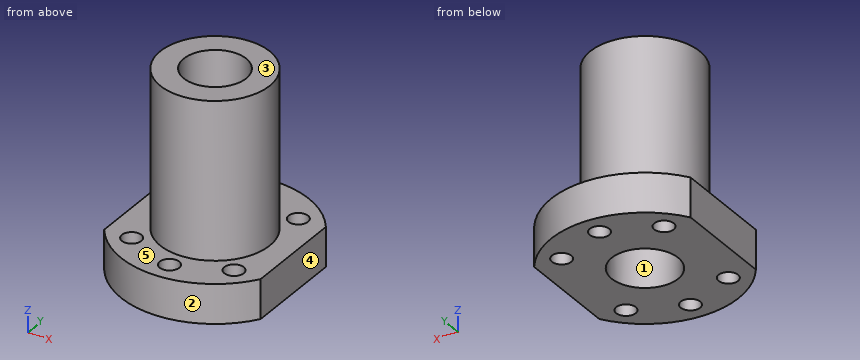
```python
from build123d import *

# Parameters (mm, degrees)
SKETCH_R      = 2.5
SKETCH_R_2    = 8.5
PAD_DEPTH     = 10
SKETCH001_R   = 14
SKETCH001_R_2 = 8
PAD001_DEPTH  = 40


with BuildPart() as part:
    # Sketch → Pad (new body)
    with BuildSketch(Plane.XY):
        with BuildLine():
            ThreePointArc((20, 13.266499), (0, 24), (-20, 13.266499))
            Line((-20, 13.266499), (-20, -13.266499))
            ThreePointArc((-20, -13.266499), (0, -24), (20, -13.266499))
            Line((20, 13.266499), (20, -13.266499))
        make_face()
        with Locations((0, 18.5)):
            Circle(SKETCH_R, mode=Mode.SUBTRACT)
        with Locations((0, -18.5)):
            Circle(SKETCH_R, mode=Mode.SUBTRACT)
        Circle(SKETCH_R_2, mode=Mode.SUBTRACT)
        with Locations((-13.081476, 13.081475)):
            Circle(SKETCH_R, mode=Mode.SUBTRACT)
        with Locations((-13.081476, -13.081475)):
            Circle(SKETCH_R, mode=Mode.SUBTRACT)
        with Locations((13.081476, -13.081475)):
            Circle(SKETCH_R, mode=Mode.SUBTRACT)
        with Locations((13.081476, 13.081475)):
            Circle(SKETCH_R, mode=Mode.SUBTRACT)
    extrude(amount=PAD_DEPTH)

    # Sketch001 → Pad001 (new body)
    with BuildSketch(Plane.XY.offset(10)):
        Circle(SKETCH001_R)
        Circle(SKETCH001_R_2, mode=Mode.SUBTRACT)
    extrude(amount=PAD001_DEPTH)


solid = part.part
```
Can you work these out from the model? Positions are in its coordinate system, mm. Face numbers are marked on the shaded views. A direction names the side the tool comes from. Give positions to 0.01 mm unless a question says otherwise; leave off trailing zeros. Loops run counter-clockwise (first coordinate to the right, second up) from the corner with the lowest first, then second, coordinate; pieces in that order, holes last. Notation, with made-up numbers: M -9,57 L 31,57 A21 ccw 31,64 Z; hole C 17.25,-4.5 d7. An arc over 180 degrees is marked long. One line per item, written item: value.
(1) I need wall thicknesses on line 1 (Y direction, x = 0, z = 33.5); line 2 (Z direction, x = 17.5, y = -15); line 3 (X direction, y = -17, z = 7). Which ranges of each line are inside material? Lowest first, please.
Returned:
line 1: -14 to -8, 8 to 14
line 2: 0 to 10
line 3: -16.94 to -2, 2 to 16.94
(2) Suppose I cut it at D-D on z = 41.5. List the corners of the cut face in (x, y) for me.
Returned:
outline: C 0,0 d28; hole C 0,0 d16
(3) Suppose I cut it at A-A on y = 0. List the corners of the cut face in (x, z) for me.
Returned:
outline: M -20,0 L -8.5,0 L -8.5,10 L -8,10 L -8,50 L -14,50 L -14,10 L -20,10 Z; M 8,10 L 8.5,10 L 8.5,0 L 20,0 L 20,10 L 14,10 L 14,50 L 8,50 Z
(4) We'd pull the mould along X, two halves only. Please class the marked faces 1, 2 and 3: released by +X, released by -X, zero draft, split by the parting line, or undercut.
Returned:
face 1: undercut
face 2: split by the parting line
face 3: zero draft
(5) Suppose I cut it at B-B on x = 0. List the corners of the cut face in (y, z) for me.
Returned:
outline: M -24,0 L -21,0 L -21,10 L -24,10 Z; M -16,0 L -8.5,0 L -8.5,10 L -8,10 L -8,50 L -14,50 L -14,10 L -16,10 Z; M 8,10 L 8.5,10 L 8.5,0 L 16,0 L 16,10 L 14,10 L 14,50 L 8,50 Z; M 21,0 L 24,0 L 24,10 L 21,10 Z
(6) Suppose I cut it at C-C on z = 7. List the corners of the cut face in (x, y) for me, plus the area to 3 significant figures.
Returned:
outline: M -20,-13.27 A24 ccw 20,-13.27 L 20,13.27 A24 ccw -20,13.27 Z; hole C -13.08,-13.08 d5; hole C -13.08,13.08 d5; hole C 0,0 d17; hole C 0,-18.5 d5; hole C 0,18.5 d5; hole C 13.08,-13.08 d5; hole C 13.08,13.08 d5
area: 1,320 mm^2
(7) Will these pins go through, and if not, where does the flat tip stop? pin 1 (3 mm diameter, centred on y = 8, z = 41.5, fed in from -X); pin 2 (3 mm diameter, centred on x = 13.08, y = 13.08, fed in from +Z); pin 3 (2 mm diameter, centred on x = -15, y = 2, fed in from -Z); pin 4 (4 mm diameter, centred on x = -6.5, z = 10, fed in from -Y).
Returned:
pin 1: x = -12.4
pin 2: through
pin 3: z = 0
pin 4: y = -23.57
(8) Which directions (+Z, -Z, +X, -X, +Y, -Y) give clear straight access to the entire face, cutting with the end or side of a thin tool? Please do the marked faces 4 and 5.
Returned:
face 4: +Z, -Z, +X, +Y, -Y
face 5: +Z
